```python
from build123d import *

# Parameters (mm, degrees)
SKETCH1_R            = 355.5
SKETCH1_R_2          = 295
BOSS_EXTRUDE1_DEPTH  = 10
BOSS_EXTRUDE2_DEPTH  = 10
FILLET1_R            = 20
CUT_EXTRUDE2_DEPTH   = 10
FILLET1_OF_MIRROR1_R = 20
CUT_EXTRUDE3_DEPTH   = 10


with BuildPart() as part:
    # Sketch1 → Boss-Extrude1 (new body)
    with BuildSketch(Plane(origin=(0, 0, 0), x_dir=(1, 0, 0), z_dir=(0, 1, 0))):
        with Locations(Location((0, 0, 0), (0, 0, 270))):
            Circle(SKETCH1_R)
        with Locations(Location((0, 0, 0), (0, 0, 270))):
            Circle(SKETCH1_R_2, mode=Mode.SUBTRACT)
    extrude(amount=BOSS_EXTRUDE1_DEPTH)

    # Sketch2 → Boss-Extrude2 (add)
    with BuildSketch(Plane(origin=(0, 10, 0), x_dir=(1, 0, 0), z_dir=(0, 1, 0))):
        with BuildLine():
            Line((-245.283583567, -262.746957418), (-201.307169156, -215.639568833))
            ThreePointArc((-201.307169156, -215.639568833), (-222.262433031, -193.970128791), (-240.896902392, -170.27531359))
            Line((-240.896902392, -170.27531359), (-290.301182374, -205.196182987))
            Line((-290.301182374, -205.196182987), (-281.950699468, -245.840512698))
            Line((-281.950699468, -245.840512698), (-279.584698805, -257.356554597))
            ThreePointArc((-279.584698805, -257.356554597), (-276.977549571, -260.160406353), (-274.342282872, -262.937847843))
            ThreePointArc((-274.342282872, -262.937847843), (-259.771835552, -269.098582225), (-245.283583567, -262.746957418))
        make_face()
    boss_extrude2 = extrude(amount=-BOSS_EXTRUDE2_DEPTH)

    # Fillet1
    fillet1_edges = [part.edges().sort_by_distance(p)[0] for p in [
        (-242.592198763, 5, 259.863954983),
        (-290.301182374, 5, 205.196182987),
    ]]
    fillet(fillet1_edges, radius=FILLET1_R)

    # Sketch5 → Cut-Extrude2 (cut)
    with BuildSketch(Plane(origin=(27.612671151, -84.821098534, 134.399234523), x_dir=(0.9852397845422893, 0.0913606537099085, -0.14476117541924585), z_dir=(0.17117992567781853, -0.5258335661753164, 0.8331845496216823))):
        Polygon((-283.235912451, 130.899924333), (-284.869220227, 115.781445421), (-336.691704543, 117.064133397), (-330.542349464, 147.835610422), (-311.799599221, 145.810758591), (-281.973151258, 142.588492009), align=None)
    extrude(amount=-CUT_EXTRUDE2_DEPTH, mode=Mode.SUBTRACT)

    # Mirror1: Boss-Extrude2 across plane
    add(boss_extrude2.mirror(Plane.XY))

    # Fillet1 of Mirror1
    fillet1_of_mirror1_edges = [part.edges().sort_by_distance(p)[0] for p in [
        (-242.592198763, 5, -259.863954983),
        (-290.301182374, 5, -205.196182987),
    ]]
    fillet(fillet1_of_mirror1_edges, radius=FILLET1_OF_MIRROR1_R)

    # Sketch7 → Cut-Extrude3 (cut)
    with BuildSketch(Plane(origin=(21.951425264, -85.580716552, -106.844235968), x_dir=(0.9873859847265816, 0.0989832733999036, 0.12357681316719149), z_dir=(-0.1583316682332344, 0.6172782613106412, 0.7706481888305408))):
        Polygon((-278.02290676, 157.72118356), (-276.013481271, 173.565711271), (-305.775097923, 177.340121727), (-307.784523411, 161.495594016), (-310.409727388, 140.795589263), (-280.648110736, 137.021178806), align=None)
    extrude(amount=-CUT_EXTRUDE3_DEPTH, mode=Mode.SUBTRACT)


solid = part.part
```
Model file for the job. Use its own axes, mm. Coordinates: 2 decimals unless noted, no trailing zeros. Write each loop counter-clockwise with the first axis right and the second up, starting at its lowest first coordinate (ties: lowest second). Pieces come first, ordered by that corner, then holes. Notation, with made-up numbers: (10.5, 25) - (30.5, 25) arc R22 ccw to (30.5, 62) - close; hole circle Ø7 at (31.5, 88). An arc over 180 degrees is marked (long way). Use a Markdown table: item, result. Add a question column.
Item 1: Band-saw the part on A-A, the plane z = 0. Write the cut outline in (x, y).
Item 2: Drill centre lines: line 1 along X through (y, z) = (4.5, 0); line 2 along X through (y, z) = (8.5, -186). Where is each one in solid material? Low to high.
Item 3: Band-saw the part on B-B, the plane x = 0. Write the cut outline in (y, z), and give its area (3 significant figures).
Item 4: Two-plate mould, pull along Z, no slides. Class faces 1 (the face through (355.32, 4.93, 11.33)), 2 (the face through (-265, 10, 133)): pulls with the +Z half, pulls with the -Z half, needs draft (parallel to the pull), parting line crosses it, or undercut.
Item 5: Drop flat-ended pins along their axis: pin 1 (5 mm diameter, centred on x = 226.5, y = 6.5, fed in from +Z); pin 2 (5 mm diameter, centred on y = 3.5, z = 270.5, fed in from +X); pin 3 (3 mm diameter, centred on x = 107.5, y = 8, fed in from +Z). Give the stop position or say it passes through.
A:
| question | item | result |
|---|---|---|
| 1 | outline | (-355.5, 0) - (-295, 0) - (-295, 10) - (-355.5, 10) - close; (295, 0) - (355.5, 0) - (355.5, 10) - (295, 10) - close |
| 2 | line 1 | x = -355.5 to -295, 295 to 355.5 |
| 2 | line 2 | x = -302.96 to -228.97, 228.97 to 302.96 |
| 3 | outline | (0, -355.5) - (10, -355.5) - (10, -295) - (0, -295) - close; (0, 295) - (10, 295) - (10, 355.5) - (0, 355.5) - close |
| 3 | area | 1,210 mm² |
| 4 | face 1 | parting line crosses it |
| 4 | face 2 | needs draft |
| 5 | pin 1 | stops at z = 276.05 |
| 5 | pin 2 | stops at x = 233.57 |
| 5 | pin 3 | stops at z = 339.33 |
